For this review, use the dimensioned drawing (mm, ordinates from the lowest corner) and the shaded views. Give positions to 0.01 mm unless a question says otherwise; leave off trailing zeros. Write each loop counter-clockwise with the first axis right and the second up, starting at its lowest first coordinate (ties: lowest second). Pieces come first, ordered by that corner, then holes.
1) We need section B-B on z = 5. Give the boundary of the cut face in (x, y).
2) We need section A-A on y = 9. Give the boundary of the cut face in (x, z), and give its area (3 significant figures).
3) Wall thickness on line 1 along Z through (x, y) = (37, 5); line 2 along X through (y, z) = (1, 4.5); line 3 along Y through (x, z) = (19.5, 6.25): over which ranges is each line inside the solid? List them lowest first.
4) Draft analysis for pull direction X (two halves, no side actions). For the marked faces 1, 2 and 3, state which applies: pulls with the +X half, pulls with the -X half, needs draft (parallel to the pull), parting line crosses it, or undercut.
5) We need section D-D on x = 22.5. Give the boundary of the cut face in (y, z), and give its area (3 significant figures).
6) For P1, Ø4, axis at x = 17, z = 8.5, coming from the +Y side; P2, Ø3, axis at x = 13.5, y = 6, coming from the -Z side; P3, Ø2, axis at x = 15.5, z = 4.5, coming from the +Y side, all flat-tipped, find the tip position at first contact; note any pin that passes through.
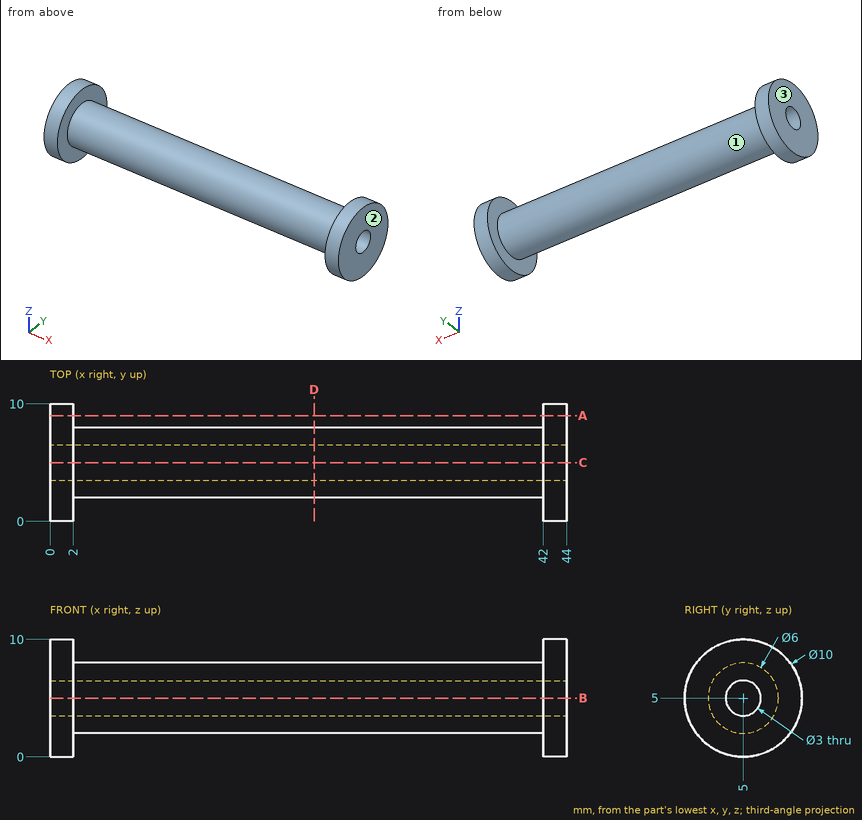
Results list:
1. outline: (0, 0) - (2, 0) - (2, 2) - (42, 2) - (42, 0) - (44, 0) - (44, 3.5) - (0, 3.5) - close; (0, 6.5) - (44, 6.5) - (44, 10) - (42, 10) - (42, 8) - (2, 8) - (2, 10) - (0, 10) - close
2. outline: (0, 2) - (2, 2) - (2, 8) - (0, 8) - close; (42, 2) - (44, 2) - (44, 8) - (42, 8) - close
2. area: 24.0 mm2
3. line 1: z = 2 to 3.5, 6.5 to 8
3. line 2: x = 0 to 2, 42 to 44
3. line 3: y = 2.27 to 4.17, 5.83 to 7.73
4. face 1: undercut
4. face 2: pulls with the +X half
4. face 3: pulls with the -X half
5. outline: circle Ø6 at (5, 5); hole circle Ø3 at (5, 5)
5. area: 21.2 mm2
6. P1: stops at y = 7.6
6. P2: stops at z = 2
6. P3: stops at y = 8
